Geometry check sheet. Reference: the model listing, model coordinates, mm. Round coordinates to 2 decimals unless told otherwise and drop trailing zeros. Order: outer loops, then holes, each group sorted by start corner. A loop starts at its lowest first (then second) coordinate and runs counter-clockwise, first axis right, second up. Notation, with made-up numbers: (1, 27) -> (48, 27) arc R27 ccw to (48, 66) -> close; hole circle Ø7 at (29.5, 5.25). An arc over 180 degrees is marked (long way). Use a Markdown table: item, result. Add a question column.
Item 1: Sectioned sample at B-B, the plane z = 2.5. Record the cut outline in (x, y), and give its area (3 significant figures).
Item 2: Gauge pin test, flat ends, axial feed: pin 1 Ø8 at (x, y) = (-51.5, 20) entering from -Z; pin 2 Ø5 at (x, y) = (-51, 20) entering from +Z. Record the tip position at first contact, or that the pin passes through.
Item 3: Material ranges on probe 1 along Y at (x, z) = (-51, 4.2); probe 2 along X at (y, z) = (-20.5, 4); probe 3 along X at (y, z) = (3, 4.5), recorded low to high. Write a range as [from, to].
Item 4: Sectioned sample at C-C, the plane y = -20. Record the cut outline in (x, z), and give its area (3 significant figures).
Item 5: Sectioned sample at A-A, the plane x = -51. Record the cut outline in (y, z), and give its area (4 significant figures).
from build123d import *

# Parameters (mm, degrees)
F0_W     = 150
F0_H     = 90
F0_R     = 5
F0_R_2   = 2.75
F1_DEPTH = 10
F2_DEPTH = 5.5


with BuildPart() as f1:
    # F0 (on Top) → F1 (new body)
    with BuildSketch(Plane.XY):
        Rectangle(F0_W, F0_H)
        with Locations((-51, -20)):
            Circle(F0_R, mode=Mode.SUBTRACT)
        with Locations((-51, 20)):
            Circle(F0_R, mode=Mode.SUBTRACT)
        with Locations((59, 0)):
            Circle(F0_R, mode=Mode.SUBTRACT)
        with Locations((-51, 20)):
            Circle(F0_R)
        with Locations((-51, 20)):
            Circle(F0_R_2, mode=Mode.SUBTRACT)
        with Locations((-51, -20)):
            Circle(F0_R)
        with Locations((-51, -20)):
            Circle(F0_R_2, mode=Mode.SUBTRACT)
        with Locations((59, 0)):
            Circle(F0_R)
        with Locations((59, 0)):
            Circle(F0_R_2, mode=Mode.SUBTRACT)
    extrude(amount=F1_DEPTH)

    # F0 (on Top) → F2 (cut)
    with BuildSketch(Plane.XY):
        with Locations((-51, -20)):
            Circle(F0_R)
        with Locations((-51, -20)):
            Circle(F0_R_2, mode=Mode.SUBTRACT)
        with Locations((-51, 20)):
            Circle(F0_R)
        with Locations((-51, 20)):
            Circle(F0_R_2, mode=Mode.SUBTRACT)
        with Locations((59, 0)):
            Circle(F0_R)
        with Locations((59, 0)):
            Circle(F0_R_2, mode=Mode.SUBTRACT)
    extrude(amount=F2_DEPTH, mode=Mode.SUBTRACT)


solid = f1.part
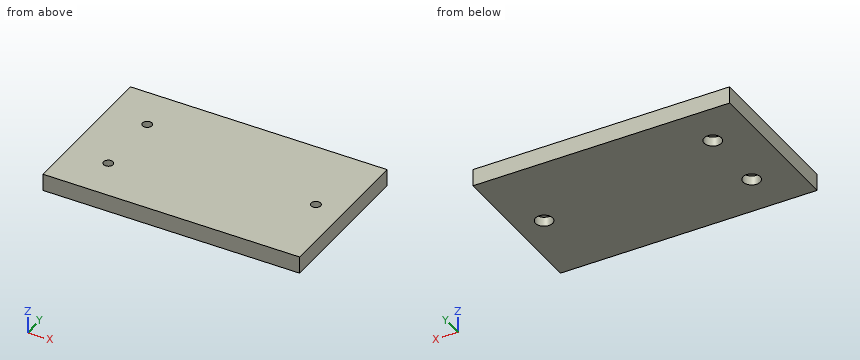
Found:
| question | item | result |
|---|---|---|
| 1 | outline | (-75, -45) -> (75, -45) -> (75, 45) -> (-75, 45) -> close; hole circle Ø10 at (-51, -20); hole circle Ø10 at (-51, 20); hole circle Ø10 at (59, 0) |
| 1 | area | 13,300 mm2 |
| 2 | pin 1 | stops at z = 5.5 |
| 2 | pin 2 | passes through |
| 3 | probe 1 | y = [-45, -25], [-15, 15], [25, 45] |
| 3 | probe 2 | x = [-75, -55.97], [-46.03, 75] |
| 3 | probe 3 | x = [-75, 55], [63, 75] |
| 4 | outline | (-75, 0) -> (-56, 0) -> (-56, 5.5) -> (-53.75, 5.5) -> (-53.75, 10) -> (-75, 10) -> close; (-48.25, 5.5) -> (-46, 5.5) -> (-46, 0) -> (75, 0) -> (75, 10) -> (-48.25, 10) -> close |
| 4 | area | 1,420 mm2 |
| 5 | outline | (-45, 0) -> (-25, 0) -> (-25, 5.5) -> (-22.75, 5.5) -> (-22.75, 10) -> (-45, 10) -> close; (-17.25, 5.5) -> (-15, 5.5) -> (-15, 0) -> (15, 0) -> (15, 5.5) -> (17.25, 5.5) -> (17.25, 10) -> (-17.25, 10) -> close; (22.75, 5.5) -> (25, 5.5) -> (25, 0) -> (45, 0) -> (45, 10) -> (22.75, 10) -> close |
| 5 | area | 740.5 mm2 |
